The drawing under review shows one solid part. Ordinate dimensions are in mm from its lowest x, y, z. Round coordinates to 2 decimals unless told otherwise and drop trailing zeros. Write each loop counter-clockwise with the first axis right and the second up, starting at its lowest first coordinate (ties: lowest second). Pieces come first, ordered by that corner, then holes.
Item 1: To check wall thickness, follow L1, parallel to X at y = 6, z = 1.8; L2, parallel to X at y = 15.5, z = 0.55 (1 decimal); L3, parallel to X at y = 31.5, z = 1.55 (1 decimal). State the ranges of each line that lie inside material, in increasing order.
Item 2: Add section C-C (y = 17.5). Give the boundary of the cut face in (x, z).
Item 3: Add section A-A (y = 8). Give the boundary of the cut face in (x, z).
Item 4: Add section B-B (z = 2.4). State how many separate pieces and enclosed holes the cut face has, plus the area to 3 significant figures.
Item 5: Clearance check with a flat-ended pin moving along its axis: pin 1 Ø1.5 at (y, z) = (8, 1) entering from -X. State where the tip first meets the part, or that it passes through.
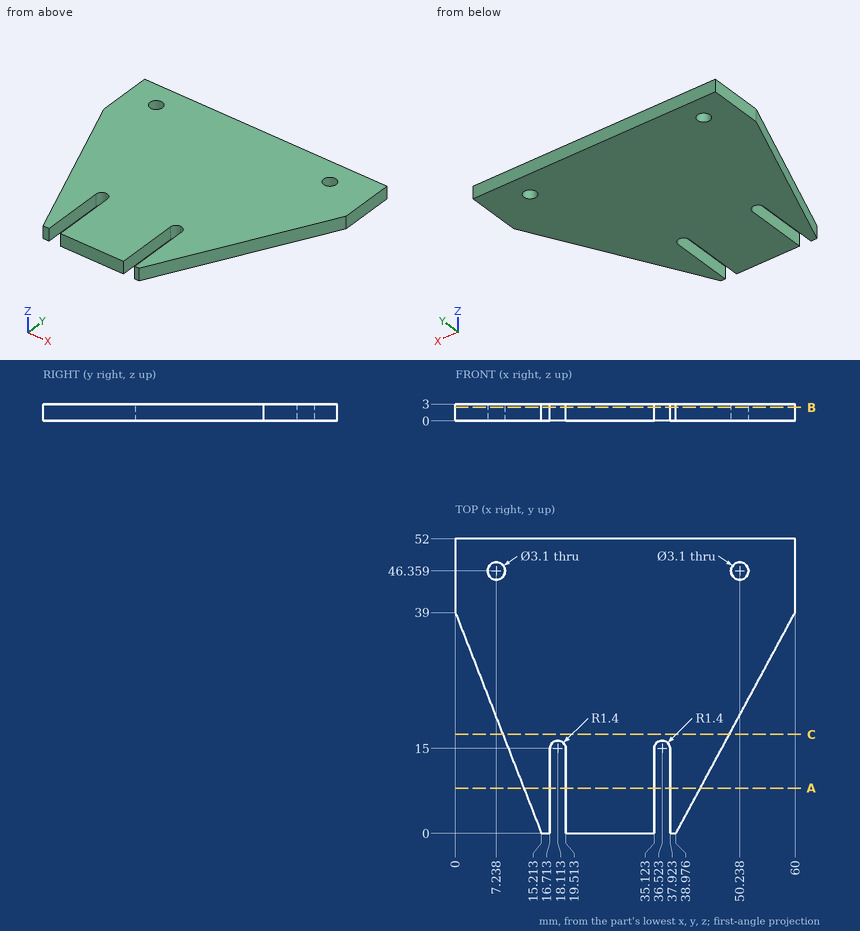
Numbers:
1. L1: x = 12.87 to 16.71, 19.51 to 35.12, 37.92 to 42.21
1. L2: x = 9.2 to 16.8, 19.4 to 35.2, 37.8 to 47.3
1. L3: x = 2.9 to 56
2. outline: (8.39, 0) - (48.41, 0) - (48.41, 3) - (8.39, 3) - close
3. outline: (12.09, 0) - (16.71, 0) - (16.71, 3) - (12.09, 3) - close; (19.51, 0) - (35.12, 0) - (35.12, 3) - (19.51, 3) - close; (37.92, 0) - (43.29, 0) - (43.29, 3) - (37.92, 3) - close
4. separate pieces: 1
4. enclosed holes: 2
4. area: 2,310 mm2
5. pin 1: stops at x = 11.8
